Can you work these out from the drawing? Everything is in mm from the part's minimum corner. Coordinates: 2 decimals unless noted, no trailing zeros. Order: outer loops, then holes, each group sorted by start corner. A loop starts at its lowest first (then second) coordinate and runs counter-clockwise, first axis right, second up. Notation, with made-up numbers: (63, 22) -> (84, 22) arc R6 ccw to (84, 26) -> close; hole circle Ø6 at (63, 30). An arc over 180 degrees is marked (long way). Return JSON: item names as keys, results as strings. Group by question number.
1) If I drill on probe 1 along Z at (x, y) = (14.5, 4.5); probe 2 along Y at (x, z) = (50, 9); probe 3 along X at (y, z) = (4.75, 4.5), over which ranges is the centre line in solid material (lowest first)? Write a range as from..to.
2) For pin 1 (3 mm diameter, centred on x = 45.5, z = 52.5, fed in from -Y); pin 2 (1.8 mm diameter, centred on x = 50, y = 5, fed in from +Z), each with a flat end and sliding along its axis, tell me the tip position at first contact or that it passes through.
3) If we section it at A-A, the plane z = 21.5: Please give me the cut outline in (x, y), then the cut area to 3 significant figures.
4) If we section it at C-C, the plane y = 5: Please give me the cut outline in (x, z), then the cut area to 3 significant figures.
5) If we section it at B-B, the plane x = 24: Please give me the cut outline in (y, z), then the cut area to 3 significant figures.
6) If we section it at D-D, the plane z = 47: Please give me the cut outline in (x, y), then the cut area to 3 significant figures.
7) Thinking about a two-plate mould opening in X: for the marked faces 1, 2, 3 and 4, which applies, +X half, -X half, draft (parallel to the pull), parting line (faces both ways), or undercut?
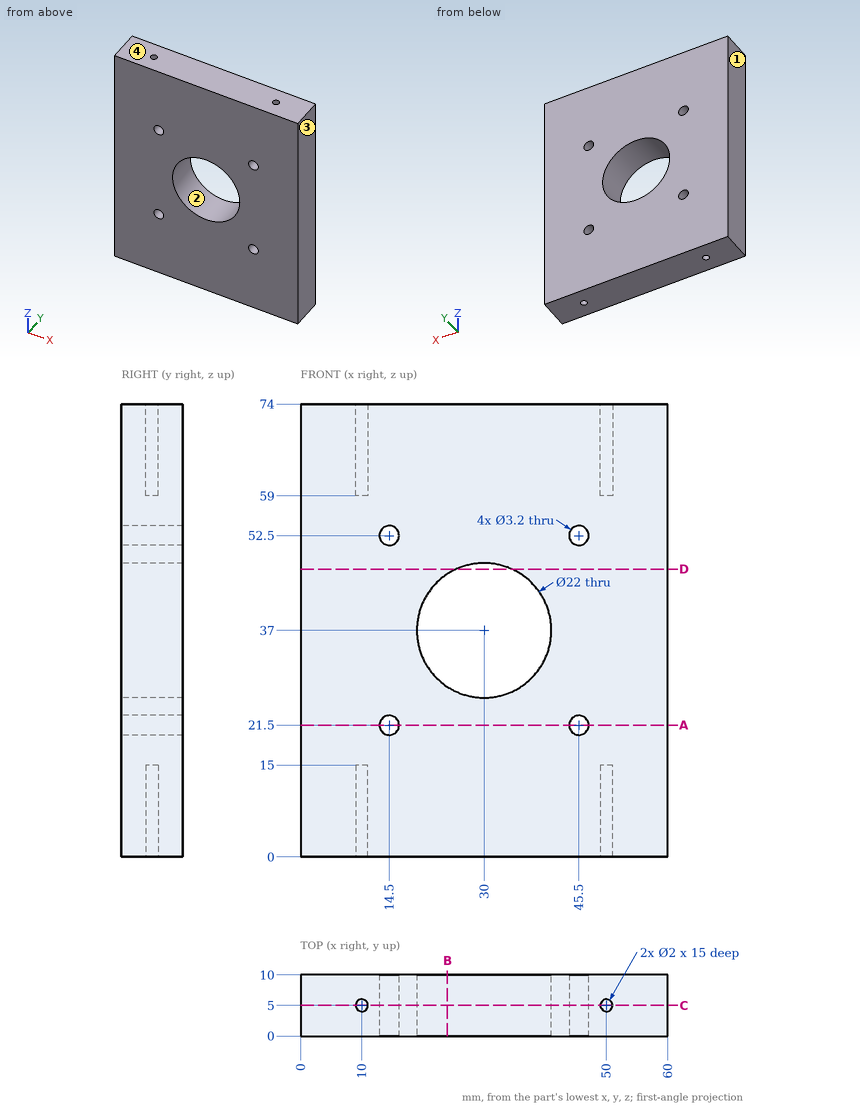
Result sheet:
{
 "1": {"probe 1": "z = 0..19.9, 23.1..50.9, 54.1..74", "probe 2": "y = 0..4, 6..10", "probe 3": "x = 0..9.03, 10.97..49.03, 50.97..60"},
 "2": {"pin 1": "passes through", "pin 2": "stops at z = 59"},
 "3": {"outline": "(0, 0) -> (12.9, 0) -> (12.9, 10) -> (0, 10) -> close; (16.1, 0) -> (43.9, 0) -> (43.9, 10) -> (16.1, 10) -> close; (47.1, 0) -> (60, 0) -> (60, 10) -> (47.1, 10) -> close", "area": "536 mm2"},
 "4": {"outline": "(0, 0) -> (9, 0) -> (9, 15) -> (11, 15) -> (11, 0) -> (49, 0) -> (49, 15) -> (51, 15) -> (51, 0) -> (60, 0) -> (60, 74) -> (51, 74) -> (51, 59) -> (49, 59) -> (49, 74) -> (11, 74) -> (11, 59) -> (9, 59) -> (9, 74) -> (0, 74) -> close; hole circle Ø3.2 at (14.5, 21.5); hole circle Ø3.2 at (14.5, 52.5); hole circle Ø22 at (30, 37); hole circle Ø3.2 at (45.5, 21.5); hole circle Ø3.2 at (45.5, 52.5)", "area": "3,910 mm2"},
 "5": {"outline": "(0, 0) -> (10, 0) -> (10, 27.78) -> (0, 27.78) -> close; (0, 46.22) -> (10, 46.22) -> (10, 74) -> (0, 74) -> close", "area": "556 mm2"},
 "6": {"outline": "(0, 0) -> (25.42, 0) -> (25.42, 10) -> (0, 10) -> close; (34.58, 0) -> (60, 0) -> (60, 10) -> (34.58, 10) -> close", "area": "508 mm2"},
 "7": {"face 1": "-X half", "face 2": "undercut", "face 3": "+X half", "face 4": "draft"}
}
